Geometry check sheet. Reference: the model listing, model coordinates, mm. Face numbers are marked on the shaded views. A direction names the side the tool comes from. Round coordinates to 2 decimals unless told otherwise and drop trailing zeros. Write each loop counter-clockwise with the first axis right and the second up, starting at its lowest first coordinate (ties: lowest second). Pieces come first, ordered by that corner, then holes. Notation, with made-up numbers: (33.25, 5) - (79.25, 5) arc R30 cw to (79.25, 40) - close; hole circle Ø9 at (78, -10.5). An arc over 180 degrees is marked (long way). Return JSON: item names as keys, results as strings.
Autodesk Inventor part; units mm, degrees
ref_plane "YZ Plane" through (0, 0, 0) normal (1, 0, 0) x (0, 1, 0)
ref_plane "XZ Plane" through (0, 0, 0) normal (0, 1, 0) x (-1, 0, 0)
ref_plane "XY Plane" through (0, 0, 0) normal (0, 0, 1) x (1, 0, 0)
sketch "Sketch1" plane through (0, 0, 0) normal (0, 0, 1) x (1, 0, 0)
  circle A0 centre (0, 0) radius 50
  dimension "d0" = 100
extrude "Extrusion1" add sketch "Sketch1" against normal blind 175
sketch "Sketch2" plane through (0, 0, 0) normal (0, 0, 1) x (1, 0, 0)
  line L0 (94.5, 57.9363) -> (94.5, -57.9363)
  line L1 (94.5, -57.9363) -> (-50, -57.9363)
  line L2 (-50, -57.9363) -> (-50, 57.9363)
  line L3 (-50, 57.9363) -> (94.5, 57.9363)
  circle A0 centre (0, 0) radius 50
  point P0 (94.5, 0)
  dimension "d3" = 144.5
  dimension "d4" = 115.8726
extrude "Extrusion2" add sketch "Sketch2" along normal blind 20 contours A0 | L0 L1 L2 L3
sketch "Sketch3" plane through (0, 0, 20) normal (0, 0, 1) x (1, 0, 0)
  arc A0 (-6, 13.7477) -> (-6, -13.7477) centre (0, 0) ccw
  arc A1 (36, -32.078) -> (36, 32.078) centre (50, 0) ccw
  line L0 (-6, 13.7477) -> (36, 32.078)
  line L1 (-6, -13.7477) -> (36, -32.078)
  dimension "d8" = 30
  dimension "d9" = 70
extrude "Extrusion3" add sketch "Sketch3" along normal blind 10
sketch "Sketch4" plane through (0, 0, 30) normal (0, 0, 1) x (1, 0, 0)
  arc A0 (36, -32.078) -> (36, 32.078) centre (50, 0) ccw
  circle A1 centre (50, 0) radius 20
  point P0 (0, 0)
  dimension "d12" = 40
extrude "Extrusion4" add sketch "Sketch4" along normal blind 10
sketch "Sketch5" plane through (50, 0, 40) normal (0, 0, 1) x (1, 0, 0)
  circle A0 centre (-50, 0) radius 50
  circle A1 centre (0, 0) radius 10
  point P0 (-100, 0)
  dimension "d15" = 20
extrude "Extrusion5" add sketch "Sketch5" along normal blind 30 contours A0 A1 | A0 A1 picked at (-3.2709, -1.921) picked at (2.9235, -2.6438)
sketch "Sketch6" plane through (50, 0, 70) normal (0, 0, 1) x (1, 0, 0)
  circle A0 centre (0, 0) radius 25
  circle A1 centre (0, 18) radius 3.75
  circle A2 centre (-15.5885, 9) radius 3.75
  circle A3 centre (-15.5885, -9) radius 3.75
  circle A4 centre (0, -18) radius 3.75
  circle A5 centre (15.5885, -9) radius 3.75
  circle A6 centre (15.5885, 9) radius 3.75
  point P0 (-50, 0)
  dimension "d18" = 50
  dimension "d19" = 7.5
  dimension "d20" = 18
  dimension "d23" = 360
extrude "Extrusion6" add sketch "Sketch6" along normal blind 5
properties part number "drivemotors"
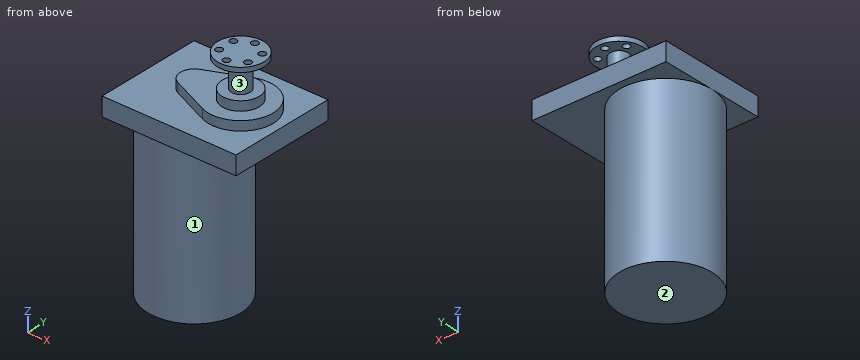
(1) Gauge pin test, flat ends, axial feed: pin 1 (3 mm diameter, centred on y = -29.5, z = -11.5, fed in from +X); pin 2 (8.5 mm diameter, centred on x = 65.59, y = -9, fed in from -Z); pin 3 (10 mm diameter, centred on x = 65.59, y = 9, fed in from +Z); pin 4 (5 mm diameter, centred on y = -34.5, z = -138.5, fed in from -X). Record the tip position at first contact, or that the pin passes through.
Response values:
{"pin 1": "stops at x = 41.42", "pin 2": "stops at z = 0", "pin 3": "stops at z = 75", "pin 4": "stops at x = -38.42"}
(2) Section check B-B, the plane x = -10. Enter the section's corners in (y, z), plus the area to 3 significant figures.
Response values:
{"outline": "(-57.94, 0) - (-48.99, 0) - (-48.99, -175) - (48.99, -175) - (48.99, 0) - (57.94, 0) - (57.94, 20) - (11.18, 20) - (11.18, 30) - (-11.18, 30) - (-11.18, 20) - (-57.94, 20) - close", "area": "19,700 mm^2"}
(3) Section check A-A, the plane y = -40. Enter the section's corners in (x, z), plus the area to 3 significant figures.
Response values:
{"outline": "(-50, 0) - (-30, 0) - (-30, -175) - (30, -175) - (30, 0) - (94.5, 0) - (94.5, 20) - (-50, 20) - close", "area": "13,400 mm^2"}
(4) Section check C-C, the plane z = -145.5. Enter the section's corners in (x, y), plus the area to 3 significant figures.
Response values:
{"outline": "circle Ø100 at (0, 0)", "area": "7,850 mm^2"}
(5) Section check D-D, the plane x = 57. Enter the section's corners in (y, z) (3 decimals).
Response values:
{"outline": "(-57.936, 0) - (57.936, 0) - (57.936, 20) - (34.293, 20) - (34.293, 30) - (18.735, 30) - (18.735, 40) - (7.141, 40) - (7.141, 70) - (24, 70) - (24, 75) - (-24, 75) - (-24, 70) - (-7.141, 70) - (-7.141, 40) - (-18.735, 40) - (-18.735, 30) - (-34.293, 30) - (-34.293, 20) - (-57.936, 20) - close"}
(6) Material ranges on line 1 along Y through (x, z) = (50, 72); line 2 along Z through (x, y) = (35.5, -15.5); line 3 along Z through (x, y) = (-41, -18.5), recorded low to high. Write a range as [from, to].
Response values:
{"line 1": "y = [-25, -21.75], [-14.25, 14.25], [21.75, 25]", "line 2": "z = [-175, 30], [70, 75]", "line 3": "z = [-175, 20]"}
(7) Access from +Z, -Z, +X, -X, +Y, -Y to the whole of each face (thin tool, end or side, straight path). Record for the marked faces 1, 2 and 3.
Response values:
{"face 1": "-Z", "face 2": "-Z, +X, -X, +Y, -Y", "face 3": "none"}
